Design review of the part built by this model. Coordinates are the model's own, in mm. A direction names the side the tool comes from. Give positions to 0.01 mm unless a question says otherwise; leave off trailing zeros. Order: outer loops, then holes, each group sorted by start corner. A loop starts at its lowest first (then second) coordinate and runs counter-clockwise, first axis right, second up.
```python
from build123d import *

# Parameters (mm, degrees)
BOSS_EXTRUDE1_START        = -4
BOSS_EXTRUDE1_DEPTH        = 4
BOSS_EXTRUDE1_DRAFT        = 7
CUT_EXTRUDE1_DEPTH         = 2
FILLET1_R                  = 2
CIRPATTERN1_COUNT          = 8
FILLET1_OF_CIRPATTERN1_R   = 2
M4X0_7_TAPPED_HOLE1_D      = 3.3
SKETCH9_R                  = 17.5
BOSS_EXTRUDE2_DEPTH        = 3
FILLET2_R                  = 1.5
F_14_0_14_DIAMETER_HOLE1_D = 14


with BuildPart() as part:
    # Sketch2 → Boss-Extrude1 (with draft: the straight prism first)
    with BuildSketch(Plane.XY.offset(BOSS_EXTRUDE1_START)):
        with BuildLine():
            ThreePointArc((-22.599988577, 34.208778352), (-29.7710089, 35.479706812), (-29.76462331, 28.19693599))
            ThreePointArc((-29.76462331, 28.19693599), (-40.960735586, 1.79391757), (-32.115758696, -25.486820975))
            ThreePointArc((-32.115758696, -25.486820975), (-32.70368863, -32.70368863), (-25.486820975, -32.115758696))
            ThreePointArc((-25.486820975, -32.115758696), (0, -41), (25.486820975, -32.115758696))
            ThreePointArc((25.486820975, -32.115758696), (32.70368863, -32.70368863), (32.115758696, -25.486820975))
            ThreePointArc((32.115758696, -25.486820975), (40.960735586, 1.79391757), (29.76462331, 28.19693599))
            ThreePointArc((29.76462331, 28.19693599), (29.7710089, 35.479706812), (22.599988577, 34.208778352))
            ThreePointArc((22.599988577, 34.208778352), (16.520796809, 37.524169182), (9.970370305, 39.769230769))
            ThreePointArc((9.970370305, 39.769230769), (0, 49), (-9.970370305, 39.769230769))
            ThreePointArc((-9.970370305, 39.769230769), (-16.520796809, 37.524169182), (-22.599988577, 34.208778352))
        make_face()
    extrude(amount=BOSS_EXTRUDE1_DEPTH)
    # Boss-Extrude1: the draft: its side faces are tilted about the plane it starts from
    boss_extrude1_sides = [part.faces().sort_by_distance(p)[0] for p in [
        (-16.520796809, 37.524169182, -2),
        (-29.7710089, 35.479706812, -2),
        (-40.960735586, 1.79391757, -2),
        (-32.70368863, -32.70368863, -2),
        (0, -41, -2),
        (32.70368863, -32.70368863, -2),
        (40.960735586, 1.79391757, -2),
        (29.7710089, 35.479706812, -2),
        (16.520796809, 37.524169182, -2),
        (0, 49, -2),
    ]]
    draft(boss_extrude1_sides, Plane.XY.offset(BOSS_EXTRUDE1_START), BOSS_EXTRUDE1_DRAFT)

    # Sketch4 → Cut-Extrude1 (cut)
    with BuildSketch(Plane.XY):
        with BuildLine():
            Line((-13.389488178, -11.268167834), (-25.786658635, -23.665338291))
            ThreePointArc((-25.786658635, -23.665338291), (-32.335783638, -13.393920133), (-34.96784237, -1.5))
            Line((-34.96784237, -1.5), (-17.435595774, -1.5))
            ThreePointArc((-17.435595774, -1.5), (-16.167891819, -6.696960066), (-13.389488178, -11.268167834))
        make_face()
    cut_extrude1 = extrude(amount=-CUT_EXTRUDE1_DEPTH, mode=Mode.SUBTRACT)

    # Fillet1
    fillet1_edges = [part.edges().sort_by_distance(p)[0] for p in [
        (-17.435595774, -1.5, -1),
        (-13.389488178, -11.268167834, -1),
        (-25.786658635, -23.665338291, -1),
        (-34.96784237, -1.5, -1),
    ]]
    fillet(fillet1_edges, radius=FILLET1_R)

    # CirPattern1: Cut-Extrude1 ×8 about axis
    cirpattern1_axis = Axis((0, 0, 0), (0, 0, 1))
    for i in range(1, CIRPATTERN1_COUNT):
        add(cut_extrude1.rotate(cirpattern1_axis, i * 360 / CIRPATTERN1_COUNT), mode=Mode.SUBTRACT)

    # Fillet1 of CirPattern1
    fillet1_of_cirpattern1_edges = [part.edges().sort_by_distance(p)[0] for p in [
        (-11.268167834, -13.389488178, -1),
        (-1.5, -17.435595774, -1),
        (-1.5, -34.96784237, -1),
        (-23.665338291, -25.786658635, -1),
        (1.5, -17.435595774, -1),
        (11.268167834, -13.389488178, -1),
        (23.665338291, -25.786658635, -1),
        (1.5, -34.96784237, -1),
        (13.389488178, -11.268167834, -1),
        (17.435595774, -1.5, -1),
        (34.96784237, -1.5, -1),
        (25.786658635, -23.665338291, -1),
        (17.435595774, 1.5, -1),
        (13.389488178, 11.268167834, -1),
        (25.786658635, 23.665338291, -1),
        (34.96784237, 1.5, -1),
        (11.268167834, 13.389488178, -1),
        (1.5, 17.435595774, -1),
        (1.5, 34.96784237, -1),
        (23.665338291, 25.786658635, -1),
        (-1.5, 17.435595774, -1),
        (-11.268167834, 13.389488178, -1),
        (-23.665338291, 25.786658635, -1),
        (-1.5, 34.96784237, -1),
        (-13.389488178, 11.268167834, -1),
        (-17.435595774, 1.5, -1),
        (-34.96784237, 1.5, -1),
        (-25.786658635, 23.665338291, -1),
    ]]
    fillet(fillet1_of_cirpattern1_edges, radius=FILLET1_OF_CIRPATTERN1_R)

    # M4x0.7 Tapped Hole1 (through all)
    with Locations(Plane(origin=(0, 0, -4), x_dir=(-1, 0, 0), z_dir=(0, 0, -1))):
        with Locations((26.717767754, 31.840995707), (29.344931419, -29.344931419), (-29.344931419, -29.344931419), (-26.717767754, 31.840995707)):
            Hole(M4X0_7_TAPPED_HOLE1_D / 2)

    # Sketch9 → Boss-Extrude2 (add)
    with BuildSketch(Plane.XY):
        Circle(SKETCH9_R)
    extrude(amount=BOSS_EXTRUDE2_DEPTH)

    # Fillet2
    fillet2_edges = [part.edges().sort_by_distance(p)[0] for p in [
        (-17.5, 0, 3),
    ]]
    fillet(fillet2_edges, radius=FILLET2_R)

    # Ø14.0 (14) Diameter Hole1 (through all)
    with Locations(Plane.XY.offset(3)):
        with Locations((0, 0)):
            Hole(F_14_0_14_DIAMETER_HOLE1_D / 2)


solid = part.part
```
1. For line 1 along Y through (x, z) = (29.5, -0.75); line 2 along X through (y, z) = (-21, -1.75); line 3 along Y through (x, z) = (-29, -1.5), list the stretches that pass through material, from the lowest coordinate up.
Recorded:
line 1: y = -33.69 to -30.99, -27.7 to -18.83, -1.5 to 1.5, 18.83 to 27.9, 28.5 to 35.19
line 2: x = -34.89 to -28, -23.12 to -18.88, -1.5 to 1.5, 18.88 to 23.12, 28 to 34.89
line 3: y = -33.77 to -30.96, -27.73 to -19.6, -1.5 to 1.5, 19.6 to 35.65
2. For pin 1 (1 mm diameter, centred on x = -9.5, z = 1.5, fed in from +Y); pin 2 (1.6 mm diameter, centred on y = -27, z = -1, fed in from -X); pin 3 (16.5 mm diameter, centred on x = -15.5, y = -28, fed in from +Z); pin 4 (2 mm diameter, centred on x = 29.34, y = -29.34, fed in from +Z), all flat-tipped, find the tip position at first contact; note any pin that passes through.
Recorded:
pin 1: stops at y = 15.01
pin 2: stops at x = -33.46
pin 3: stops at z = 0
pin 4: passes through
3. Machinability: for faces 4 (the face through (30.92, -28.85, -1.97)), 5 (the face through (-1.5, -26, -1)), which of the approach directions +Z, -Z, +X, -X, +Y, -Y give a long, thin tool a straight path to every point of the face, cutting with its end or side? Answer none if there is none.
Recorded:
face 4: +Z, -Z
face 5: +Z
4. Draft analysis for pull direction Y (two halves, no side actions). For faces 1 (the face through (-25.761, 22.726, -1.014)), 2 (the face through (-0.39, -40.7, -1.58)), 3 (the face through (26, 1.5, -1)), state which applies: pulls with the +Y half, pulls with the -Y half, needs draft (parallel to the pull), parting line crosses it, or undercut.
Recorded:
face 1: undercut
face 2: pulls with the -Y half
face 3: undercut
5. Take a section at B-B (y = 0). State the section outline as (x, z) points.
Recorded:
outline: (-41, -4) - (-7, -4) - (-7, 3) - (-16, 3) arc R1.5 ccw to (-17.5, 1.5) - (-17.5, 0) - (-40.51, 0) - close; (7, -4) - (41, -4) - (40.51, 0) - (17.5, 0) - (17.5, 1.5) arc R1.5 ccw to (16, 3) - (7, 3) - close
6. Take a section at C-C (z = -3). State the section outline as (x, y) points.
Recorded:
outline: (-31.94, -25.51) arc R4.63 ccw (long way) to (-25.51, -31.94) arc R40.88 ccw to (25.51, -31.94) arc R4.63 ccw (long way) to (31.94, -25.51) arc R40.88 ccw to (29.58, 28.21) arc R4.63 ccw (long way) to (22.64, 34.03) arc R40.88 ccw to (9.85, 39.67) arc R9.88 ccw to (-9.85, 39.67) arc R40.88 ccw to (-22.64, 34.03) arc R4.63 ccw (long way) to (-29.58, 28.21) arc R40.88 ccw to start; hole circle Ø3.3 at (-29.34, -29.34); hole circle Ø3.3 at (-26.72, 31.84); hole circle Ø14 at (0, 0); hole circle Ø3.3 at (26.72, 31.84); hole circle Ø3.3 at (29.34, -29.34)
7. Take a section at A-A (x = 0). State the section outline as (y, z) points.
Recorded:
outline: (-41, -4) - (-7, -4) - (-7, 3) - (-16, 3) arc R1.5 ccw to (-17.5, 1.5) - (-17.5, 0) - (-40.51, 0) - close; (7, -4) - (49, -4) - (48.51, 0) - (17.5, 0) - (17.5, 1.5) arc R1.5 ccw to (16, 3) - (7, 3) - close
